Can you work these out from the model? Positions are in its coordinate system, mm. A direction names the side the tool comes from. Give positions to 0.01 mm unless a question says otherwise; leave off trailing zeros. Loops run counter-clockwise (first coordinate to the right, second up) from the corner with the lowest first, then second, coordinate; pieces in that order, holes last. Notation, with made-up numbers: M -28,42.25 L 0,42.25 A27 ccw 0,60.25 Z; hole C 75.5,73.25 d8. An arc over 180 degrees is marked long. Answer as a JSON object with one key per item and string values.
```python
from build123d import *

# Parameters (mm, degrees)
FILLET1_R                                            = 5
CSK_FOR_M12_HEX_SOCKET_COUNTERSUNK_CAP_S_D           = 14
CSK_FOR_M12_HEX_SOCKET_COUNTERSUNK_CAP_S_CSINK_D     = 26
CSK_FOR_M12_HEX_SOCKET_COUNTERSUNK_CAP_S_CSINK_ANGLE = 90
CSK_FOR_M6_HEX_SOCKET_COUNTERSUNK_CAP_SC_D           = 6.5
CSK_FOR_M6_HEX_SOCKET_COUNTERSUNK_CAP_SC_CSINK_D     = 7.5
CSK_FOR_M6_HEX_SOCKET_COUNTERSUNK_CAP_SC_CSINK_ANGLE = 90
CIRPATTERN1_COUNT                                    = 6


with BuildPart() as part:
    # Sketch1 → Revolve1 (revolve)
    with BuildSketch(Plane.XY):
        Polygon((0, 0), (-28, 0), (-28, 35), (-23, 35), (-23, 47.5), (-18, 47.5), (-18, 14), (0, 14), align=None)
    revolve(axis=Axis((0, 0, 0), (-1, 0, 0)))

    # Fillet1
    fillet1_edges = [part.edges().sort_by_distance(p)[0] for p in [
        (-18, -14, 0),
    ]]
    fillet(fillet1_edges, radius=FILLET1_R)

    # CSK for M12 Hex Socket Countersunk Cap Screw1 (through all)
    with Locations(Plane.ZY.offset(28)):
        with Locations((0, 0)):
            CounterSinkHole(CSK_FOR_M12_HEX_SOCKET_COUNTERSUNK_CAP_S_D / 2, CSK_FOR_M12_HEX_SOCKET_COUNTERSUNK_CAP_S_CSINK_D / 2, counter_sink_angle=CSK_FOR_M12_HEX_SOCKET_COUNTERSUNK_CAP_S_CSINK_ANGLE)

    # CSK for M6 Hex Socket Countersunk Cap Screw1 (through all)
    with Locations(Plane(origin=(-18, 0, 0), x_dir=(0, 0, -1), z_dir=(1, 0, 0))):
        with Locations((-40, 0)):
            csk_for_m6_hex_socket_countersunk_cap_sc = CounterSinkHole(CSK_FOR_M6_HEX_SOCKET_COUNTERSUNK_CAP_SC_D / 2, CSK_FOR_M6_HEX_SOCKET_COUNTERSUNK_CAP_SC_CSINK_D / 2, counter_sink_angle=CSK_FOR_M6_HEX_SOCKET_COUNTERSUNK_CAP_SC_CSINK_ANGLE)

    # CirPattern1: CSK for M6 Hex Socket Countersunk Cap Screw1 ×6 about axis
    cirpattern1_axis = Axis((0, 0, 0), (1, 0, 0))
    for i in range(1, CIRPATTERN1_COUNT):
        add(csk_for_m6_hex_socket_countersunk_cap_sc.rotate(cirpattern1_axis, i * 360 / CIRPATTERN1_COUNT), mode=Mode.SUBTRACT)


solid = part.part
```
1) If we mould it in two halves opening along Z, with no side actions, what happens to faces 1 (the flat face through (-28, 0, 15)), 2 (the cylindrical face through (-10.846, -2.681, -6.466)), 3 (the cylindrical face through (-25, -28, 21))? For each: +Z half, -Z half, draft (parallel to the pull), parting line (faces both ways), or undercut.
Answer list:
{"face 1": "draft", "face 2": "undercut", "face 3": "parting line"}
2) Suppose I cut it at A-A, the plane y = 0. Give the number of separate pieces and of enclosed holes in the cut face, and give its area (3 significant figures).
Answer list:
{"separate pieces": "4", "enclosed holes": "0", "area": "846 mm^2"}
3) Suppose I cut it at C-C, the plane y = 20.5. Write out the boundary of the cut face in (x, z), and give its area (3 significant figures).
Answer list:
{"outline": "M -28,-28.37 L -23,-28.37 L -23,-42.85 L -18,-42.85 L -18,42.85 L -23,42.85 L -23,28.37 L -28,28.37 Z", "area": "712 mm^2"}
4) For faces 4 (the cylindrical face through (-20.782, 31.901, 18.253)), 5 (the flat face through (-23, -20.9, -28.4)), 6 (the flat face through (-18, 20, -1)), which set-ups out of +Z, -Z, +X, -X, +Y, -Y let a thin tool reach every point of the face, with its end or its side?
Answer list:
{"face 4": "+X, -X", "face 5": "-X", "face 6": "+X"}
5) Please list where these lines run through material, in increasing order: line 1 along Z through (x, y) = (-19.65, 0); line 2 along Y through (x, z) = (-9.75, 0); line 3 along Y through (x, z) = (-21.35, -20). Write a range as from..to.
Answer list:
{"line 1": "-47.5..-43.25, -36.75..-7, 7..36.75, 43.25..47.5", "line 2": "-14..-7, 7..14", "line 3": "-43.08..-37.89, -31.39..31.39, 37.89..43.08"}
6) Will these pins go through, and if not, where does the flat tip stop? pin 1 Ø8.5 at (y, z) = (0, -40) entering from +X; pin 2 Ø6 at (x, z) = (-13, 3.5) entering from +Y; pin 3 Ø1 at (x, y) = (-15, -4) entering from +Z.
Answer list:
{"pin 1": "x = -18", "pin 2": "y = 14.67", "pin 3": "z = 14.14"}
7) Suppose I cut it at B-B, the plane x = -5.5. Write out the boundary of the cut face in (y, z), and give its area (3 significant figures).
Answer list:
{"outline": "C 0,0 d28; hole C 0,0 d14", "area": "462 mm^2"}
